```python
from build123d import *

# Parameters (mm, degrees)
FILLET1_R   = 0.25
HEX_2_DEPTH = 3


with BuildPart() as part:
    # BodySke → Base-Revolve (revolve)
    with BuildSketch(Plane.XY):
        Polygon((0, 0), (0, 4.4), (0.6, 5), (6, 5), (6, 3), (30.4455, 3), (31, 2.4455), (31, 0), align=None)
    revolve(axis=Axis((-31.75, 0, 0), (1, 0, 0)))

    # Fillet1
    fillet1_edges = [part.edges().sort_by_distance(p)[0] for p in [
        (6, -3, 0),
    ]]
    fillet(fillet1_edges, radius=FILLET1_R)

    # Sketch2 → Hex-PreBroach (revolve, cut)
    with BuildSketch(Plane.XY):
        Polygon((0, 2.542), (3, 2.542), (4.467624384, 0), (0, 0), align=None)
    revolve(axis=Axis((0, 0, 0), (1, 0, 0)), mode=Mode.SUBTRACT)

    # Sketch3 → Hex 2 (cut)
    with BuildSketch(Plane(origin=(0, 0, 0), x_dir=(0, 0.5, 0.866025404), z_dir=(-1, 0, 0))):
        Polygon((1.467624384, 2.542), (-1.467624384, 2.542), (-2.935248769, 0), (-1.467624384, -2.542), (1.467624384, -2.542), (2.935248769, 0), align=None)
    extrude(amount=-HEX_2_DEPTH, mode=Mode.SUBTRACT)


solid = part.part
```
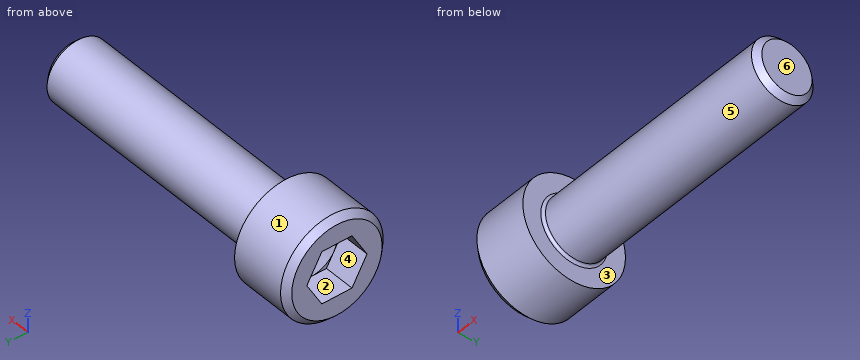
For this review, take the finished solid that the model builds, in its own axes (mm). Face numbers are marked on the shaded views. A direction names the side the tool comes from. Coordinates: 2 decimals unless noted, no trailing zeros. Loops run counter-clockwise (first coordinate to the right, second up) from the corner with the lowest first, then second, coordinate; pieces in that order, holes last. Notation, with made-up numbers: (-31.5, 32) -> (-13.5, 32) arc R34 cw to (-13.5, 67) -> close; hole circle Ø3 at (43.5, 32). An arc over 180 degrees is marked (long way). Return JSON: item names as keys, results as strings. Group by question number.
(1) Consider section A-A, the plane x = 9. Give the boundary of the cut face in (y, z).
(2) For pin 1 Ø0.8 at (y, z) = (-2.5, -0.5) entering from -X; pin 2 Ø1 at (y, z) = (-2, 4) entering from +X, all flat-tipped, find the tip position at first contact; note any pin that passes through.
(3) Mouldability with a two-part tool opening along Z and no side actions: class the marked faces 1, 2 and 3 as pulls with the +Z half, pulls with the -Z half, needs draft (parallel to the pull), parting line crosses it, or undercut.
(4) To check wall thickness, follow L1, parallel to X at y = -1.5, z = 1.5; L2, parallel to X at y = 4, z = 0.5; L3, parallel to Y at x = 20, z = 0.25. State the ranges of each line that lie inside material, in increasing order.
(5) Tool access review of the marked faces 4, 5 and 6: name each direction out of +Z, -Z, +X, -X, +Y, -Y from which nothing blocks a thin tool from reaching the whole face with its end or side.
Results below:
{
 "1": {"outline": "circle Ø6 at (0, 0)"},
 "2": {"pin 1": "stops at x = 0", "pin 2": "stops at x = 6"},
 "3": {"face 1": "parting line crosses it", "face 2": "undercut", "face 3": "needs draft"},
 "4": {"L1": "x = 3.24 to 31", "L2": "x = 0 to 6", "L3": "y = -2.99 to 2.99"},
 "5": {"face 4": "-X", "face 5": "+X", "face 6": "+Z, -Z, +X, +Y, -Y"}
}
